Autodesk Inventor part; units mm, degrees
ref_plane "YZ Plane" through (0, 0, 0) normal (1, 0, 0) x (0, 1, 0)
ref_plane "XZ Plane" through (0, 0, 0) normal (0, 1, 0) x (-1, 0, 0)
ref_plane "XY Plane" through (0, 0, 0) normal (0, 0, 1) x (1, 0, 0)
sketch "Sketch1" plane through (0, 0, 0) normal (0, 0, 1) x (1, 0, 0)
  line L0 (0, 0) -> (0, 50.8)
  line L1 (0, 0) -> (50.8, 0)
  line L2 (50.8, 4.7625) -> (4.7625, 4.7625)
  line L3 (4.7625, 4.7625) -> (4.7625, 50.8)
  line L4 (50.8, 0) -> (50.8, 4.7625)
  line L5 (0, 50.8) -> (4.7625, 50.8)
  line L6 (4.7625, 50.8) -> (50.8, 4.7625)
  line L7 (4.7625, 44.0648) -> (44.0648, 4.7625)
  dimension "d0" = 50.8
  dimension "d1" = 50.8
  dimension "d2" = 4.7625
  dimension "d3" = 4.7625
extrude "Extrusion1" add sketch "Sketch1" along normal blind 22.225 contours L0 L5 L3 L2 L4 L1 | L6 L2 L7 L3
sketch "Sketch2" plane through (0, 0, 0) normal (0, -1, 0) x (1, 0, 0)
  line L0 (0, 0) -> (0, 22.225)
  line L1 (0, 14.1605) -> (50.8, 14.1605)
  line L2 (50.8, 0) -> (50.8, 22.225)
  line L3 (50.8, 8.0645) -> (0, 8.0645)
  line L4 (0, 0) -> (50.8, 0)
  line L5 (50.8, 14.1605) -> (50.8, 8.0645)
  line L6 (0, 14.1605) -> (0, 8.0645)
  dimension "d6" = 6.096
  dimension "d7" = 8.0645
extrude "Extrusion2" add sketch "Sketch2" along normal blind 3.175 contours L0 L1 L2 L3
properties part number "Triangle Bracket"
Verification items for the finished model (mm, model axes). A direction names the side the tool comes from. Round coordinates to 2 decimals unless told otherwise and drop trailing zeros. Write each loop counter-clockwise with the first axis right and the second up, starting at its lowest first coordinate (ties: lowest second). Pieces come first, ordered by that corner, then holes.
1. Section check B-B on x = 22. Enter the section's corners in (y, z) (1 decimal), plus the area to 3 significant figures.
2. Scan lines: L1, parallel to Y at x = 17, z = 18; L2, parallel to Y at x = 26, z = 13.75 (1 decimal); L3, parallel to X at y = 38, z = 14.5. Record each from-to range of solid material in increasing order.
3. Access from +Z, -Z, +X, -X, +Y, -Y to the whole of each face (thin tool, end or side, straight path). Record for faces 1 (the flat face through (24.14, 24.69, 10.96)), 2 (the flat face through (25, -2, 14.16)), 3 (the flat face through (2, 50.8, 11)), 4 (the flat face through (26, -2, 8.065)).
4. Section check C-C on y = 19.5. Enter the section's corners in (x, z) (1 decimal).
5. Gauge pin test, flat ends, axial feed: P1, Ø5, axis at y = 5, z = 13, coming from the -X side; P2, Ø1.6, axis at x = 31.5, y = -2, coming from the +Z side; P3, Ø1, axis at x = 35, y = -1.5, coming from the -Z side; P4, Ø6.5, axis at x = 33.5, z = 2, coming from the -Y side. Record the tip position at first contact, or that the pin passes through.
6. Draft check along Y on faces 5 (the flat face through (25, 4.762, 11)), 6 (the flat face through (25, 0, 4)), 7 (the flat face through (4.762, 24, 11)), 8 (the flat face through (0, 23, 11)). Enter one of: +Y half, -Y half, draft (parallel to the pull), parting line (faces both ways), or undercut.
7. Section check A-A on z = 3. Enter the section's corners in (x, y), plus the area to 3 significant figures.
8. Section check D-D on z = 11.75. Enter the section's corners in (x, y) (1 decimal), plus the area to 3 significant figures.
Answer:
1. outline: (-3.2, 8.1) - (0, 8.1) - (0, 0) - (4.8, 0) - (4.8, 22.2) - (0, 22.2) - (0, 14.2) - (-3.2, 14.2) - close; (26.8, 0) - (33.6, 0) - (33.6, 22.2) - (26.8, 22.2) - close
1. area: 275 mm2
2. L1: y = 0 to 4.76, 31.83 to 38.56
2. L2: y = -3.2 to 4.8, 22.8 to 29.6
2. L3: x = 0 to 4.76, 10.83 to 17.56
3. face 1: +Z, -Z
3. face 2: +Z, +X, -X, -Y
3. face 3: +Z, -Z, +X, -X, +Y
3. face 4: -Z, +X, -X, -Y
4. outline: (0, 0) - (4.8, 0) - (4.8, 22.2) - (0, 22.2) - close; (29.3, 0) - (36.1, 0) - (36.1, 22.2) - (29.3, 22.2) - close
5. P1: stops at x = 0
5. P2: stops at z = 14.16
5. P3: stops at z = 8.06
5. P4: stops at y = 0
6. face 5: undercut
6. face 6: -Y half
6. face 7: undercut
6. face 8: draft
7. outline: (0, 0) - (50.8, 0) - (50.8, 4.76) - (4.76, 50.8) - (0, 50.8) - close; hole (4.76, 4.76) - (44.06, 4.76) - (4.76, 44.06) - close
7. area: 749 mm2
8. outline: (0, -3.2) - (50.8, -3.2) - (50.8, 4.8) - (4.8, 50.8) - (0, 50.8) - close; hole (4.8, 4.8) - (44.1, 4.8) - (4.8, 44.1) - close
8. area: 910 mm2
